from build123d import *

# Parameters (mm, degrees)
SKETCH1_W           = 82
SKETCH1_H           = 82
SKETCH1_H_2         = 10
SKETCH1_W_2         = 10
BOSS_EXTRUDE1_DEPTH = 20
SKETCH1_3_W         = 10
SKETCH1_3_H         = 82
SKETCH1_3_H_2       = 10
SKETCH1_3_W_2       = 82
BOSS_EXTRUDE2_DEPTH = 34
FILLET1_R           = 10
CUT_EXTRUDE2_DEPTH  = 10
CUT_EXTRUDE3_DEPTH  = 10
FILLET2_R           = 5
FILLET3_R           = 2


with BuildPart() as part:
    # Sketch1 → Boss-Extrude1 (new body)
    with BuildSketch(Plane(origin=(0, 0, 0), x_dir=(1, 0, 0), z_dir=(0, 1, 0))):
        with Locations((15.533475027, -31.001062699)):
            Rectangle(SKETCH1_W, SKETCH1_H)
        with Locations((15.533475027, 14.998937301)):
            Rectangle(SKETCH1_W, SKETCH1_H_2)
        with Locations((-30.466524973, 14.998937301)):
            Rectangle(SKETCH1_W_2, SKETCH1_H_2)
        with Locations((-30.466524973, -31.001062699)):
            Rectangle(SKETCH1_W_2, SKETCH1_H)
    extrude(amount=BOSS_EXTRUDE1_DEPTH)

    # Sketch1_3 → Boss-Extrude2 (add)
    with BuildSketch(Plane(origin=(0, 0, 0), x_dir=(1, 0, 0), z_dir=(0, 1, 0))):
        with Locations((-30.466524973, -31.001062699)):
            Rectangle(SKETCH1_3_W, SKETCH1_3_H)
        with Locations((-30.466524973, 14.998937301)):
            Rectangle(SKETCH1_3_W, SKETCH1_3_H_2)
        with Locations((15.533475027, 14.998937301)):
            Rectangle(SKETCH1_3_W_2, SKETCH1_3_H_2)
    extrude(amount=BOSS_EXTRUDE2_DEPTH)

    # Fillet1
    fillet1_edges = [part.edges().sort_by_distance(p)[0] for p in [
        (56.533475027, 17, -19.998937301),
        (-35.466524973, 17, -19.998937301),
        (-35.466524973, 17, 72.001062699),
        (56.533475027, 10, 72.001062699),
    ]]
    fillet(fillet1_edges, radius=FILLET1_R)

    # Sketch5 → Cut-Extrude2 (cut)
    with BuildSketch(Plane(origin=(0, 20, 0), x_dir=(1, 0, 0), z_dir=(0, 1, 0))):
        Polygon((5.533475027, -57.001062699), (10.533475027, -57.001062699), (20.532072448, -57.001062699), (5.533475027, -47.001062699), align=None)
        Polygon((-9.466524973, -57.001062699), (0.533475027, -57.001062699), (5.533475027, -57.001062699), (5.533475027, -47.001062699), align=None)
        Polygon((0.533475027, -72.001062699), (10.533475027, -72.001062699), (10.533475027, -57.001062699), (5.533475027, -57.001062699), (0.533475027, -57.001062699), align=None)
    extrude(amount=-CUT_EXTRUDE2_DEPTH, mode=Mode.SUBTRACT)

    # Sketch6 → Cut-Extrude3 (cut)
    with BuildSketch(Plane(origin=(0, 20, 0), x_dir=(1, 0, 0), z_dir=(0, 1, 0))):
        Polygon((41.533475027, -26.001062699), (56.533475027, -26.001062699), (56.533475027, -16.001062699), (41.533475027, -16.001062699), (41.533475027, -21.001062699), align=None)
        Polygon((31.533475027, -21.001062699), (41.533475027, -21.001062699), (41.533475027, -16.001062699), (41.533475027, -6.001062699), align=None)
        Polygon((41.533475027, -36.001062699), (41.533475027, -26.001062699), (41.533475027, -21.001062699), (31.533475027, -21.001062699), align=None)
    extrude(amount=-CUT_EXTRUDE3_DEPTH, mode=Mode.SUBTRACT)

    # Fillet2
    fillet2_edges = [part.edges().sort_by_distance(p)[0] for p in [
        (31.533475027, 15, 21.001062699),
        (5.533475027, 15, 47.001062699),
    ]]
    fillet(fillet2_edges, radius=FILLET2_R)

    # Fillet3
    fillet3_edges = [part.edges().sort_by_distance(p)[0] for p in [
        (41.533475027, 15, 6.001062699),
        (41.533475027, 15, 36.001062699),
        (-9.466524973, 15, 57.001062699),
        (20.532072448, 15, 57.001062699),
    ]]
    fillet(fillet3_edges, radius=FILLET3_R)


solid = part.part
Geometry: final body of the model. Coordinates: model frame, mm. A direction names the side the tool comes from. Give positions to 0.01 mm unless a question says otherwise; leave off trailing zeros. Order: outer loops, then holes, each group sorted by start corner. A loop starts at its lowest first (then second) coordinate and runs counter-clockwise, first axis right, second up. Notation, with made-up numbers: (0, 7.25) -> (30, 7.25) arc R11 cw to (30, 18.25) -> close; hole circle Ø6 at (-33, 57). An arc over 180 degrees is marked (long way). Answer as a JSON object with one key per item and string values.
Q1. Section A-A (y = 14). Output: boundary loops of the cut face in (x, z), plus the area to 3 significant figures.
Entries:
{"outline": "(-35.47, -10) arc R10 ccw to (-25.47, -20) -> (46.53, -20) arc R10 ccw to (56.53, -10) -> (56.53, 16) -> (41.53, 16) -> (41.53, 12.61) arc R2 cw to (37.87, 11.5) -> (33.38, 18.23) arc R5 cw to (33.38, 23.77) -> (37.87, 30.5) arc R2 cw to (41.53, 29.4) -> (41.53, 26) -> (56.53, 26) -> (56.53, 62) arc R10 ccw to (46.53, 72) -> (10.53, 72) -> (10.53, 57) -> (13.93, 57) arc R2 cw to (15.04, 53.34) -> (8.31, 48.85) arc R5 cw to (2.76, 48.85) -> (-3.97, 53.34) arc R2 cw to (-2.86, 57) -> (0.53, 57) -> (0.53, 72) -> (-25.47, 72) arc R10 ccw to (-35.47, 62) -> close", "area": "7,810 mm^2"}
Q2. First-contact query: pin 1 (24.5 mm diameter, centred on x = 8.5, z = 50, fed in from +Y); pin 2 (5 mm diameter, centred on x = 52, y = 14, fed in from +Z); pin 3 (4 mm diameter, centred on y = 25.5, z = 17.5, fed in from +X). Flat tips, straight axial feed; report the tip coordinate or a pass-through.
Entries:
{"pin 1": "stops at y = 20", "pin 2": "stops at z = 71.55", "pin 3": "stops at x = -25.47"}
Q3. Section C-C (z = 0.5). Output: boundary loops of the cut face in (x, y).
Entries:
{"outline": "(-35.47, 0) -> (56.53, 0) -> (56.53, 20) -> (-25.47, 20) -> (-25.47, 34) -> (-35.47, 34) -> close"}
Q4. Section D-D (y = 24). Output: boundary loops of the cut face in (x, z), plus the area to 3 significant figures.
Entries:
{"outline": "(-35.47, -10) arc R10 ccw to (-25.47, -20) -> (46.53, -20) arc R10 ccw to (56.53, -10) -> (-25.47, -10) -> (-25.47, 72) arc R10 ccw to (-35.47, 62) -> close", "area": "1,680 mm^2"}
Q5. Draft query along Z for faces 1 (the flat face through (-27, 34, 5)), 2 (the flat face through (49, 15, 16.001)), 3 (the flat face through (11, 17, -19.999)). Return one class per face: released by +Z, released by -Z, zero draft, split by the parting line, or undercut.
Entries:
{"face 1": "zero draft", "face 2": "undercut", "face 3": "released by -Z"}
Q6. Access query for faces 4 (the cylindrical face through (-4.764, 14.93, 55.615)), 5 (the cylindrical face through (53.682, 10.14, 68.994)), 6 (the flat face through (0.533, 15, 64)), 7 (the cylindrical face through (-32.615, 16.762, 68.994)), 8 (the flat face through (-25.467, 27, 32)). Directions: +Z, -Z, +X, -X, +Y, -Y. A direction counts if a zero-diameter tool reaches every point of the face in a straight line with its end or side. Return the directions, or none.
Entries:
{"face 4": "+Y", "face 5": "+Z, +X, +Y, -Y", "face 6": "+Z, +Y", "face 7": "+Z, -X, +Y, -Y", "face 8": "+Z, +X, +Y"}
Q7. Section B-B (x = 21.5). Output: boundary loops of the cut face in (y, z).
Entries:
{"outline": "(0, -20) -> (34, -20) -> (34, -10) -> (20, -10) -> (20, 72) -> (0, 72) -> close"}
Q8. Material intervals for probe 1 along Z at (x, y) = (45.5, 17); probe 2 along Y at (x, z) = (-20.5, 3.5); probe 3 along Y at (x, z) = (12.5, 54), sorted ascending.
Entries:
{"probe 1": "z = -20 to 16, 26 to 72", "probe 2": "y = 0 to 20", "probe 3": "y = 0 to 10"}
